Geometry check sheet. Reference: the model listing, model coordinates, mm. A direction names the side the tool comes from. Coordinates: 2 decimals unless noted, no trailing zeros. Loops run counter-clockwise (first coordinate to the right, second up) from the corner with the lowest first, then second, coordinate; pieces in that order, holes last.
from build123d import *
from build123d.topology import SkipClean

# Parameters (mm, degrees)
SKETCH1_R               = 22.5
BOSS_EXTRUDE1_DEPTH     = 3
SKETCH2_R               = 5
BOSS_EXTRUDE2_DEPTH     = 70
SKETCH3_R               = 12
BOSS_EXTRUDE3_DEPTH     = 28
FILLET1_R               = 6
SKETCH4_W               = 13.909985693
SKETCH4_H               = 20
CUT_EXTRUDE1_DEPTH      = 80.633535649
CUT_EXTRUDE1_DEPTH_BACK = 80.633535649
SKETCH8_R               = 4
CUT_EXTRUDE3_DEPTH      = 83.068568892
SKETCH10_R              = 9
SKETCH10_R_2            = 4
BOSS_EXTRUDE5_DEPTH     = 12.5


with BuildPart() as part:
    # Sketch1 → Boss-Extrude1 (new body)
    with BuildSketch(Plane(origin=(0, 0, 0), x_dir=(1, 0, 0), z_dir=(0, 1, 0))):
        with Locations(Location((0, 0, 0), (0, 0, 270))):
            Circle(SKETCH1_R)
    extrude(amount=BOSS_EXTRUDE1_DEPTH)

    # Sketch2 → Boss-Extrude2 (add)
    with BuildSketch(Plane(origin=(0, 3, 0), x_dir=(1, 0, 0), z_dir=(0, 1, 0))):
        with Locations(Location((0, 0, 0), (0, 0, 270))):
            Circle(SKETCH2_R)
    extrude(amount=BOSS_EXTRUDE2_DEPTH)

    # Sketch3 → Boss-Extrude3 (add)
    with BuildSketch(Plane.XZ):
        with Locations(Location((0, 0, 0), (0, 0, 270))):
            Circle(SKETCH3_R)
    extrude(amount=BOSS_EXTRUDE3_DEPTH)

    # Fillet1
    fillet1_edges = [part.edges().sort_by_distance(p)[0] for p in [
        (0, -28, 12),
    ]]
    fillet(fillet1_edges, radius=FILLET1_R)

    # Sketch4 → Cut-Extrude1 (cut, two sides)
    with BuildSketch(Plane(origin=(0, 0, 0), x_dir=(0, 0, -1), z_dir=(1, 0, 0))) as cut_extrude1_sk:
        with Locations((14.454992847, -18)):
            Rectangle(SKETCH4_W, SKETCH4_H)
        with Locations((-14.454992847, -18)):
            Rectangle(SKETCH4_W, SKETCH4_H)
    extrude(amount=CUT_EXTRUDE1_DEPTH, mode=Mode.SUBTRACT)
    extrude(cut_extrude1_sk.sketch, amount=-CUT_EXTRUDE1_DEPTH_BACK, mode=Mode.SUBTRACT)

    # Sketch8 → Cut-Extrude3 (cut, through all)
    with BuildSketch(Plane(origin=(0, 0, -7.5), x_dir=(-1, 0, 0), z_dir=(0, 0, -1))):
        with Locations(Location((0, -18, 0), (0, 0, 90))):
            Circle(SKETCH8_R)
    extrude(amount=-CUT_EXTRUDE3_DEPTH, mode=Mode.SUBTRACT)

    # Sketch10 → Boss-Extrude5 (add, symmetric)
    with SkipClean():  # the faces are left unmerged after this step: merging them gives an invalid solid
        with BuildSketch(Plane.XY):
            with Locations(Location((0, -18, 0), (0, 0, 270))):
                Circle(SKETCH10_R)
            with Locations((0, -18)):
                Circle(SKETCH10_R_2, mode=Mode.SUBTRACT)
        extrude(amount=BOSS_EXTRUDE5_DEPTH, both=True)


solid = part.part
1) Section check A-A on z = 10.5. Record the cut outline in (x, y), and give its area (3 significant figures).
Data:
outline: (-19.9, 0) - (-5.81, 0) - (-5.81, -8) - (5.81, -8) - (5.81, 0) - (19.9, 0) - (19.9, 3) - (-19.9, 3) - close; circle Ø18 at (0, -18); hole circle Ø8 at (0, -18)
area: 417 mm2
2) Material ranges on probe 1 along Y at (x, z) = (0, 2); probe 2 along X at (y, z) = (-18, 8.5); probe 3 along X at (y, z) = (-18, -4), recorded low to high.
Data:
probe 1: y = -28 to -22, -14 to 73
probe 2: x = -9 to -4, 4 to 9
probe 3: x = -11.31 to -4, 4 to 11.31
3) Access from +Z, -Z, +X, -X, +Y, -Y to the whole of each face (thin tool, end or side, straight path). Record for faces 1 (the flat face through (-2, -9, 7.5)), 2 (the cylindrical face through (-4.88, 37.51, -1.08)), 3 (the cylindrical face through (2.703, -26.584, -9.965)).
Data:
face 1: +Z
face 2: +Y
face 3: -Z
4) Depth check by flat-ended pin: pin 1 (6.5 mm diameter, centred on x = 0, y = -18, fed in from +Z); pin 2 (12 mm diameter, centred on x = 11, z = 17.5, fed in from +Y); pin 3 (3.5 mm diameter, centred on x = -3, z = 11, fed in from -Y); pin 4 (6 mm diameter, centred on x = -4, y = 22, fed in from -Z). Enter the tip coordinate at first touch or a pass-through.
Data:
pin 1: passes through
pin 2: stops at y = 3
pin 3: stops at y = -26.91
pin 4: stops at z = -4.9
5) Section check D-D on x = -19. Record the cut outline in (y, z), and give its area (3 significant figures).
Data:
outline: (0, -12.05) - (3, -12.05) - (3, 12.05) - (0, 12.05) - close
area: 72.3 mm2
6) Mould release check, pull along Y, two halves, no side actions. Record for faces 4 (the flat face through (-2, -22, -12.5)), 5 (the flat face through (0, -8, -9)), 6 (the flat face through (0, -28, 0)): +Y half, -Y half, draft (parallel to the pull), parting line (faces both ways), or undercut.
Data:
face 4: draft
face 5: undercut
face 6: -Y half
7) Section check B-B on y = 37. Record the cut outline in (x, z).
Data:
outline: circle Ø10 at (0, 0)
8) Section check C-C on x = 19.5. Record the cut outline in (y, z).
Data:
outline: (0, -11.22) - (3, -11.22) - (3, 11.22) - (0, 11.22) - close
